Drawing for the job (mm, zero at the part's lowest x, y, z). A direction names the side the tool comes from. Give positions to 0.01 mm unless a question says otherwise; leave off trailing zeros. Order: outer loops, then holes, each group sorted by start corner. A loop starts at its lowest first (then second) coordinate and runs counter-clockwise, first axis right, second up. Notation, with made-up numbers: (-10, -1.75) - (47, -1.75) arc R29 cw to (47, 34.25) - close; hole circle Ø5 at (66, -30.5). An arc over 180 degrees is marked (long way). One line per item, written item: value.
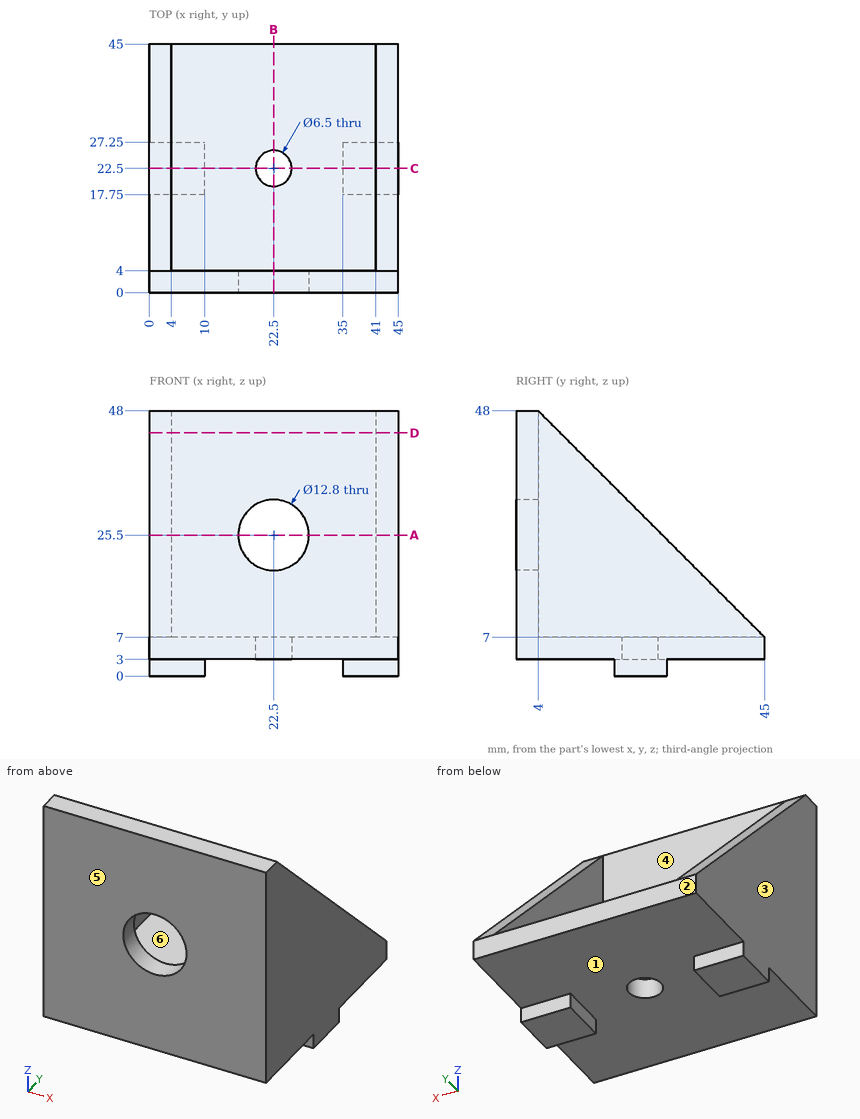
1) Cut at A-A, the plane z = 25.5. Give the cut face in (x, y).
Outcome:
outline: (0, 0) - (16.1, 0) - (16.1, 4) - (4, 4) - (4, 26.5) - (0, 26.5) - close; (28.9, 0) - (45, 0) - (45, 26.5) - (41, 26.5) - (41, 4) - (28.9, 4) - close
2) Cut at D-D, the plane z = 44. Give the cut face in (x, y), then the cut area to 3 significant figures.
Outcome:
outline: (0, 0) - (45, 0) - (45, 8) - (41, 8) - (41, 4) - (4, 4) - (4, 8) - (0, 8) - close
area: 212 mm^2
3) Which spindle directions (+Z, -Z, +X, -X, +Y, -Y) get a long thin tool onto all of the face, cutting with end or side? Do the marked faces 5 and 6. Say none if no direction does.
Outcome:
face 5: +Z, -Z, +X, -X, -Y
face 6: +Z, +Y
4) Cut at B-B, the plane x = 22.5. Give the cut face in (y, z).
Outcome:
outline: (0, 3) - (19.25, 3) - (19.25, 7) - (4, 7) - (4, 19.1) - (0, 19.1) - close; (0, 31.9) - (4, 31.9) - (4, 48) - (0, 48) - close; (25.75, 3) - (45, 3) - (45, 7) - (25.75, 7) - close
5) Pin check, flat tips, straight feed: pin 1 (12.5 mm diameter, centred on y = 33, z = 22.5, fed in from -X); pin 2 (1.5 mm diameter, centred on x = 42.5, z = 1, fed in from +Y); pin 3 (2 mm diameter, centred on x = 31.5, y = 13.5, fed in from +Z); pin 4 (12 mm diameter, centred on x = 20, y = 28.5, fed in from -Z). Stop position of each tip, or through.
Outcome:
pin 1: stops at x = 0
pin 2: stops at y = 27.25
pin 3: stops at z = 7
pin 4: stops at z = 3
6) Mould opens along X. For the marked faces 1, 2, 3 and 4 say: released by +X, released by -X, zero draft, split by the parting line, or undercut.
Outcome:
face 1: undercut
face 2: zero draft
face 3: released by -X
face 4: undercut
7) Cut at C-C, the plane y = 22.5. Give the cut face in (x, z), then the cut area to 3 significant figures.
Outcome:
outline: (0, 0) - (10, 0) - (10, 3) - (19.25, 3) - (19.25, 7) - (4, 7) - (4, 29.5) - (0, 29.5) - close; (25.75, 3) - (35, 3) - (35, 0) - (45, 0) - (45, 29.5) - (41, 29.5) - (41, 7) - (25.75, 7) - close
area: 394 mm^2
8) Drill centre lines: line 1 along Z through (x, y) = (22.5, 1.8); line 2 along X through (y, z) = (7, 13.5); line 3 along Y through (x, z) = (4.5, 25). Where is each one in solid material? Low to high. Write a range as from..to.
Outcome:
line 1: z = 3..19.1, 31.9..48
line 2: x = 0..4, 41..45
line 3: y = 0..4
